Build history of the part. All positions in model axes, mm. Round coordinates to 2 decimals unless told otherwise and drop trailing zeros. Loops run counter-clockwise (first coordinate to the right, second up) from the corner with the lowest first, then second, coordinate; pieces in that order, holes last. Notation, with made-up numbers: (55.5, -28) - (83.5, -28) arc R29 ccw to (83.5, 9) - close; hole circle Ø8 at (-34.5, 37). An arc over 180 degrees is marked (long way). Use a Markdown table: item, result.
from build123d import *

# Parameters (mm, degrees)
SKETCH_1_R      = 10
EXTRUDE_1_DEPTH = 9
SCALE_2_SCALE   = 1.2
SHELL_3_T       = -1.2


with BuildPart() as part:
    # 草图1 → 凸台-拉伸1 (new body)
    with BuildSketch(Plane.XY):
        Circle(SKETCH_1_R)
    extrude(amount=EXTRUDE_1_DEPTH)


with BuildPart() as part_1:
    # 缩放比例2: scaled about (0, 0, 0)
    add(part.part.scale(SCALE_2_SCALE))

    # 抽壳3
    shell_3_openings = [part_1.faces().sort_by_distance(p)[0] for p in [
        (0, 0, 10.8),
        (0, 0, 0),
    ]]
    offset(amount=SHELL_3_T, openings=shell_3_openings, kind=Kind.INTERSECTION)


solid = part_1.part
Q1. Cut at B-B, the plane y = 0.5. List the corners of the cut face in (x, z), plus the area to 3 significant figures.
Results found:
| item | result |
|---|---|
| outline | (-11.99, 0) - (-10.79, 0) - (-10.79, 10.8) - (-11.99, 10.8) - close; (10.79, 0) - (11.99, 0) - (11.99, 10.8) - (10.79, 10.8) - close |
| area | 25.9 mm2 |
Q2. Probe line 1 (Y direction, x = 0, z = 3.25); line 2 (X direction, y = -2.5, z = 8.5); line 3 (Y direction, x = 4.5, z = 3.25). List the from-to ranges inside material, lowest first.
Results found:
| item | result |
|---|---|
| line 1 | y = -12 to -10.8, 10.8 to 12 |
| line 2 | x = -11.74 to -10.51, 10.51 to 11.74 |
| line 3 | y = -11.12 to -9.82, 9.82 to 11.12 |
Q3. Cut at A-A, the plane x = 0. List the corners of the cut face in (y, z), plus the area to 3 significant figures.
Results found:
| item | result |
|---|---|
| outline | (-12, 0) - (-10.8, 0) - (-10.8, 10.8) - (-12, 10.8) - close; (10.8, 0) - (12, 0) - (12, 10.8) - (10.8, 10.8) - close |
| area | 25.9 mm2 |
Q4. Cut at C-C, the plane z = 7.75. List the corners of the cut face in (x, y).
Results found:
| item | result |
|---|---|
| outline | circle Ø24 at (0, 0); hole circle Ø21.6 at (0, 0) |
Q5. Drop flat-ended pins along their axis: pin 1 (4 mm diameter, centred on x = 6.5, y = 3.5, fed in from +Z); pin 2 (2 mm diameter, centred on x = 8, z = 4, fed in from +Y); pin 3 (3 mm diameter, centred on y = -2.5, z = 9.5, fed in from -X); pin 4 (3 mm diameter, centred on x = -2, z = 8.5, fed in from +Y). Give the stop position or say it passes through.
Results found:
| item | result |
|---|---|
| pin 1 | passes through |
| pin 2 | stops at y = 9.75 |
| pin 3 | stops at x = -11.96 |
| pin 4 | stops at y = 11.99 |
Q6. Pull direction Y, two halves, no side cores. Call faces 1 (the face through (-10, 5, 10.8)), 2 (the face through (-11.99, 0.53, 5.32)), 3 (the face through (-2.341, -10.543, 5.324)): pulls with the +Y half, pulls with the -Y half, needs draft (parallel to the pull), parting line crosses it, or undercut.
Results found:
| item | result |
|---|---|
| face 1 | needs draft |
| face 2 | parting line crosses it |
| face 3 | undercut |
